Design review of the part built by this model. Coordinates are the model's own, in mm. A direction names the side the tool comes from. Give positions to 0.01 mm unless a question says otherwise; leave off trailing zeros. Order: outer loops, then holes, each group sorted by start corner. A loop starts at its lowest first (then second) coordinate and runs counter-clockwise, first axis right, second up. Notation, with made-up numbers: (51.25, 23) -> (71.25, 23) arc R30 ccw to (71.25, 57) -> close; hole circle Ø4 at (66.5, -30.75). An arc over 180 degrees is marked (long way). One line per item, written item: value. Start each with the question number.
1) For pin 1 (4 mm diameter, centred on y = 130, z = 8, fed in from +X); pin 2 (3 mm diameter, centred on x = -3.5, y = -77.5, fed in from +Z), all flat-tipped, find the tip position at first contact; note any pin that passes through.
2) Consider section A-A (y = -180.5). State the section outline as (x, z) points.
3) Consider section B-B (z = -3.75). State the section outline as (x, y) points, plus the area to 3 significant figures.
4) Wall thickness on line 1 along Y through (x, z) = (-3.5, -10.85); line 2 along X through (y, z) = (-202.5, -10.15); line 3 along X through (y, z) = (-283.8, -10.65): over which ranges is each line inside the solid? List them lowest first. Write a range as from..to.
5) Consider section C-C (x = 7). State the section outline as (y, z) points.
6) Tool access review of faces 1 (the face through (2, -4, -9.5)), 2 (the face through (0, -4, -12.7)): name each direction out of +Z, -Z, +X, -X, +Y, -Y from which nothing blocks a thin tool from reaching the whole face with its end or side.
from build123d import *

# Parameters (mm, degrees)
F1_DEPTH = 291
F3_SIZE2 = 10.1
F3_SIZE  = 88
F4_SIZE2 = 25
F4_SIZE  = 9.5
F5_R     = 1.75
F6_DEPTH = 3.2
F2_R     = 1.35
F7_DEPTH = 25.401


with BuildPart() as f1:
    # F0 (on Front) → F1 (new body, symmetric)
    with BuildSketch(Plane.XZ):
        Polygon((-9.5, 12.7), (-12.7, 12.7), (-12.7, -12.7), (12.7, -12.7), (12.7, -9.5), (-9.5, -9.5), align=None)
    extrude(amount=F1_DEPTH, both=True)

    # F3
    f3_edges = [f1.edges().sort_by_distance(p)[0] for p in [
        (-11.1, -291, 12.7),
    ]]
    f3_side = f1.faces().sort_by_distance((-11.1, 0, 12.7))[0]
    chamfer(f3_edges, length=F3_SIZE, length2=F3_SIZE2, reference=f3_side)

    # F4
    f4_edges = [f1.edges().sort_by_distance(p)[0] for p in [
        (-11.1, 291, 12.7),
    ]]
    f4_side = f1.faces().sort_by_distance((-11.1, 291, 12.34079))[0]
    chamfer(f4_edges, length=F4_SIZE, length2=F4_SIZE2, reference=f4_side)

    # F5 (on face) → F6 (cut, through all)
    with BuildSketch(Plane.XY.offset(-9.5)):
        with Locations((0, -283.8)):
            Circle(F5_R)
        with Locations((0, 283.8)):
            Circle(F5_R)
    extrude(amount=-F6_DEPTH, mode=Mode.SUBTRACT)

    # F2 (on face) → F7 (cut, through all)
    with BuildSketch(Plane(origin=(0, 0, -12.7), x_dir=(1, 0, 0), z_dir=(0, 0, -1))):
        with Locations((-3.5, 77.5)):
            Circle(F2_R)
        with Locations((-3.5, -77.5)):
            Circle(F2_R)
        with Locations((-3.5, -202.5)):
            Circle(F2_R)
        with Locations((-3.5, 202.5)):
            Circle(F2_R)
    extrude(amount=-F7_DEPTH, mode=Mode.SUBTRACT)


solid = f1.part
Checked values:
1. pin 1: stops at x = -9.5
1. pin 2: stops at z = -9.5
2. outline: (-12.7, -12.7) -> (12.7, -12.7) -> (12.7, -9.5) -> (-9.5, -9.5) -> (-9.5, 12.7) -> (-12.7, 12.7) -> close
3. outline: (-12.7, -291) -> (-9.5, -291) -> (-9.5, 291) -> (-12.7, 291) -> close
3. area: 1,860 mm^2
4. line 1: y = -291..-203.85, -201.15..-78.85, -76.15..76.15, 78.85..201.15, 203.85..291
4. line 2: x = -12.7..-4.85, -2.15..12.7
4. line 3: x = -12.7..-1.75, 1.75..12.7
5. outline: (-291, -12.7) -> (291, -12.7) -> (291, -9.5) -> (-291, -9.5) -> close
6. face 1: +Z, +X, +Y, -Y
6. face 2: -Z, +X, -X, +Y, -Y
